Design review of the part built by this model. Coordinates are the model's own, in mm. Face numbers are marked on the shaded views. A direction names the side the tool comes from. Coordinates: 2 decimals unless noted, no trailing zeros. Loops run counter-clockwise (first coordinate to the right, second up) from the corner with the lowest first, then second, coordinate; pieces in that order, holes last. Notation, with made-up numbers: (83, 26) - (132, 26) arc R12 cw to (132, 45) - close; hole circle Ø8 at (50.5, 85.25). An arc over 180 degrees is marked (long way). Return JSON: item names as keys, results as strings. Group by question number.
from build123d import *

# Parameters (mm, degrees)
CROQUIS1_W              = 23
CROQUIS1_H              = 20
SALIENTE_EXTRUIR1_DEPTH = 9
CROQUIS2_W              = 6
CROQUIS2_H              = 12.95
CORTAR_EXTRUIR1_DEPTH   = 2
CROQUIS3_W              = 2.5
CROQUIS3_H              = 20
SALIENTE_EXTRUIR3_DEPTH = 15
CROQUIS4_R              = 1.85
CORTAR_EXTRUIR4_DEPTH   = 2.5
SALIENTE_EXTRUIR7_DEPTH = 2.5
CROQUIS7_W              = 10
CROQUIS7_H              = 15
CORTAR_EXTRUIR5_DEPTH   = 2.5
CROQUIS8_W              = 23
CROQUIS8_H              = 20
CORTAR_EXTRUIR6_DEPTH   = 3
CROQUIS9_W              = 2.5
CROQUIS9_H              = 10
CORTAR_EXTRUIR7_DEPTH   = 2
REDONDEO1_R             = 7
REDONDEO2_R             = 1


with BuildPart() as part:
    # Croquis1 → Saliente-Extruir1 (new body)
    with BuildSketch(Plane(origin=(0, 0, 0), x_dir=(1, 0, 0), z_dir=(0, 1, 0))):
        with Locations((11.5, -10)):
            Rectangle(CROQUIS1_W, CROQUIS1_H)
    extrude(amount=SALIENTE_EXTRUIR1_DEPTH)

    # Croquis2 → Cortar-Extruir1 (cut)
    with BuildSketch(Plane(origin=(0, 9, 0), x_dir=(1, 0, 0), z_dir=(0, 1, 0))):
        with Locations((20, -9.475)):
            Rectangle(CROQUIS2_W, CROQUIS2_H)
    extrude(amount=-CORTAR_EXTRUIR1_DEPTH, mode=Mode.SUBTRACT)

    # Croquis3 → Saliente-Extruir3 (add)
    with BuildSketch(Plane(origin=(0, 9, 0), x_dir=(1, 0, 0), z_dir=(0, 1, 0))):
        with Locations((1.25, -10)):
            Rectangle(CROQUIS3_W, CROQUIS3_H)
    extrude(amount=SALIENTE_EXTRUIR3_DEPTH)

    # Croquis4 → Cortar-Extruir4 (cut)
    with BuildSketch(Plane(origin=(2.5, 0, 0), x_dir=(0, 0, -1), z_dir=(1, 0, 0))):
        with Locations((-18, 15)):
            Circle(CROQUIS4_R)
    extrude(amount=-CORTAR_EXTRUIR4_DEPTH, mode=Mode.SUBTRACT)

    # Croquis6 → Saliente-Extruir7 (add)
    with BuildSketch(Plane(origin=(2.5, 0, 0), x_dir=(0, 0, -1), z_dir=(1, 0, 0))):
        with BuildLine():
            Line((-20, 19.418427322), (-20, 10.581572678))
            ThreePointArc((-20, 10.581572678), (-22.85, 15), (-20, 19.418427322))
        make_face()
    extrude(amount=-SALIENTE_EXTRUIR7_DEPTH)

    # Croquis7 → Cortar-Extruir5 (cut)
    with BuildSketch(Plane(origin=(2.5, 0, 0), x_dir=(0, 0, -1), z_dir=(1, 0, 0))):
        with Locations((-5, 16.5)):
            Rectangle(CROQUIS7_W, CROQUIS7_H)
    extrude(amount=-CORTAR_EXTRUIR5_DEPTH, mode=Mode.SUBTRACT)

    # Croquis8 → Cortar-Extruir6 (cut)
    with BuildSketch(Plane.XZ):
        with Locations((11.5, 10)):
            Rectangle(CROQUIS8_W, CROQUIS8_H)
    extrude(amount=-CORTAR_EXTRUIR6_DEPTH, mode=Mode.SUBTRACT)

    # Croquis9 → Cortar-Extruir7 (cut)
    with BuildSketch(Plane(origin=(0, 24, 0), x_dir=(1, 0, 0), z_dir=(0, 1, 0))):
        with Locations((1.25, -15)):
            Rectangle(CROQUIS9_W, CROQUIS9_H)
    extrude(amount=-CORTAR_EXTRUIR7_DEPTH, mode=Mode.SUBTRACT)

    # Redondeo1
    # the kernel refuses this fillet: 7 mm, written as the material it adds along each edge
    with BuildSketch(Plane(origin=(2.5, 9, 10), x_dir=(0, 0, -1), z_dir=(-1, 0, 0))) as redondeo1_piece_1:
        with BuildLine():
            CenterArc((REDONDEO1_R, -REDONDEO1_R), REDONDEO1_R, 90, 90)
            Line((0, -REDONDEO1_R), (0, 0))
            Line((0, 0), (REDONDEO1_R, 0))
        make_face()
    extrude(amount=2.5)
    with BuildSketch(Plane(origin=(2.5, 9, 10), x_dir=(1, 0, 0), z_dir=(0, 0, 1))) as redondeo1_piece_2_section:
        with BuildLine():
            CenterArc((REDONDEO1_R, REDONDEO1_R), REDONDEO1_R, 180, 90)
            Line((0, REDONDEO1_R), (0, 0))
            Line((0, 0), (REDONDEO1_R, 0))
        make_face()
    redondeo1_piece_2 = extrude(amount=10, mode=Mode.PRIVATE)
    redondeo1_piece_2 = redondeo1_piece_2 - Plane(origin=(2.5, 15, 18), x_dir=(0, 0, -1), z_dir=(1, 0, 0)) * Cylinder(1.85, 48, mode=Mode.PRIVATE)
    add(redondeo1_piece_2)
    with BuildSketch(Plane(origin=(2.5, 9, -7.5), x_dir=(1, 0, 0), z_dir=(0, 0, 1))) as redondeo1_piece_3_section:
        with BuildLine():
            CenterArc((REDONDEO1_R, REDONDEO1_R), REDONDEO1_R, 180, 90)
            Line((0, REDONDEO1_R), (0, 0))
            Line((0, 0), (REDONDEO1_R, 0))
        make_face()
    redondeo1_piece_3 = extrude(amount=45, mode=Mode.PRIVATE)
    redondeo1_piece_3 = split(redondeo1_piece_3, bisect_by=Plane(origin=(2.5, 9, 20), z_dir=(0, 0, 1)), keep=Keep.TOP, mode=Mode.PRIVATE)
    redondeo1_piece_3 = redondeo1_piece_3 & Plane(origin=(2.5, 15, 18), x_dir=(0, -0.9110159426851695, 0.4123711340206198), z_dir=(1, 0, 0)) * Cylinder(4.85, 118, mode=Mode.PRIVATE)
    add(redondeo1_piece_3)
    with BuildSketch(Plane(origin=(2.5, 9, -7.5), x_dir=(1, 0, 0), z_dir=(0, 0, 1))) as redondeo1_piece_4a_section:
        with BuildLine():
            CenterArc((REDONDEO1_R, REDONDEO1_R), REDONDEO1_R, 180, 90)
            Line((0, REDONDEO1_R), (0, 0))
            Line((0, 0), (REDONDEO1_R, 0))
        make_face()
    redondeo1_piece_4a = extrude(amount=27.5, mode=Mode.PRIVATE)
    redondeo1_piece_4a = split(redondeo1_piece_4a, bisect_by=Plane(origin=(2.5, 9, 0), z_dir=(0, 0, 1)), keep=Keep.TOP, mode=Mode.PRIVATE)
    redondeo1_piece_4a = split(redondeo1_piece_4a, bisect_by=Plane(origin=(2.5, 9, 10), z_dir=(0, 0, -1)), keep=Keep.TOP, mode=Mode.PRIVATE)
    with BuildSketch(Plane(origin=(20, 9, 10), x_dir=(0, 0, -1), z_dir=(-1, 0, 0))) as redondeo1_piece_4b_section:
        with BuildLine():
            CenterArc((REDONDEO1_R, -REDONDEO1_R), REDONDEO1_R, 90, 90)
            Line((0, -REDONDEO1_R), (0, 0))
            Line((0, 0), (REDONDEO1_R, 0))
        make_face()
    redondeo1_piece_4b = extrude(amount=20, mode=Mode.PRIVATE)
    redondeo1_piece_4b = split(redondeo1_piece_4b, bisect_by=Plane(origin=(2.5, 9, 10), z_dir=(1, 0, 0)), keep=Keep.TOP, mode=Mode.PRIVATE)
    redondeo1_piece_4b = split(redondeo1_piece_4b, bisect_by=Plane(origin=(17, 9, 10), z_dir=(-1, 0, 0)), keep=Keep.TOP, mode=Mode.PRIVATE)
    redondeo1_piece_4 = redondeo1_piece_4a & redondeo1_piece_4b
    add(redondeo1_piece_4)

    # Redondeo2
    redondeo2_edges = [part.edges().sort_by_distance(p)[0] for p in [
        (4.977657648, 10.656927883, 7.522342352),
        (0, 19, 10),
        (0, 11.050252532, 7.949747468),
        (7.147234739, 9.40723915, 20),
        (1.25, 22, 20),
        (0, 22, 15),
        (2.5, 22, 15),
        (2.5, 19, 10),
        (23, 9, 1.5),
        (23, 9, 17.975),
        (11.5, 9, 0),
        (0, 9, 1.5),
        (16.25, 9, 20),
    ]]
    fillet(redondeo2_edges, radius=REDONDEO2_R)


solid = part.part
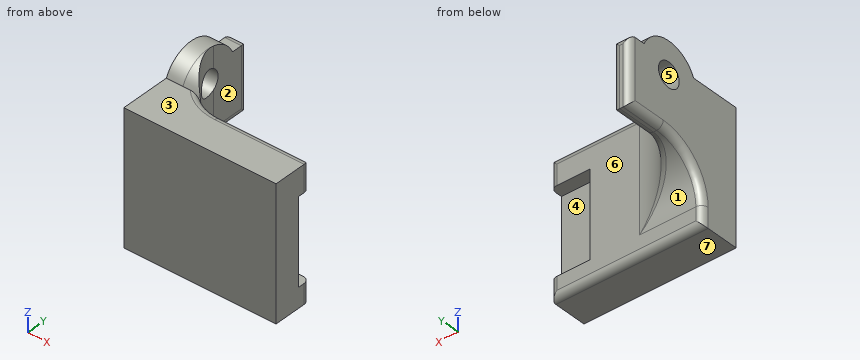
Item 1: Add section B-B (x = 20). State the section outline as (y, z) points.
Item 2: Add section A-A (z = 18). State the section outline as (x, y) points, then the cut area to 3 significant figures.
Item 3: To check wall thickness, follow line 1 (Y direction, x = 1.2, z = 18); line 2 (Y direction, x = 17, z = 17.5); line 3 (X direction, y = 7.75, z = 8.25). State the ranges of each line that lie inside material, in increasing order. Write a range as from..to.
Item 4: Add section C-C (y = 7.5). State the section outline as (x, z) points, then the cut area to 3 significant figures.
Item 5: For P1, Ø1.8, axis at x = 18.5, z = 6.5, coming from the +Y side; P2, Ø0.5, axis at x = 1.5, y = 20, coming from the +Z side; P3, Ø6, axis at x = 19.5, y = 11.5, coming from the +Z side, all flat-tipped, find the tip position at first contact; note any pin that passes through.
Item 6: Add section D-D (z = 13). State the section outline as (x, y) points.
Item 7: Draft analysis for pull direction Z (two halves, no side actions). For the marked faces 5, 6 and 7, state which applies: pulls with the +Z half, pulls with the -Z half, needs draft (parallel to the pull), parting line crosses it, or undercut.
Item 8: For the marked faces 1, 2, 3 and 4, list the 3-axis set-ups (+Z, -Z, +X, -X, +Y, -Y) from which the entire face can be reached by the end or side of a thin tool; tool diameter is ignored.
Answers below:
{
 "1": {"outline": "(3, 0) - (8, 0) arc R1 ccw to (9, 1) - (9, 3) - (7, 3) - (7, 15.95) - (9, 15.95) - (9, 19) arc R1 ccw to (8, 20) - (3, 20) - close"},
 "2": {"outline": "(0, 3) - (23, 3) - (23, 8) arc R1 ccw to (22, 9) - (9.5, 9) arc R7 cw to (3.11, 13.15) - (0, 13.15) - close; (0, 16.85) - (2.5, 16.85) - (2.5, 21) arc R1 ccw to (1.5, 22) - (1, 22) arc R1 ccw to (0, 21) - close", "area": "171 mm^2"},
 "3": {"line 1": "y = 3..13.15, 16.85..22", "line 2": "y = 3..9", "line 3": "x = 0..17"},
 "4": {"outline": "(0, 0) - (23, 0) - (23, 3) - (17, 3) - (17, 15.95) - (23, 15.95) - (23, 20) - (0, 20) - close", "area": "382 mm^2"},
 "5": {"P1": "stops at y = 7", "P2": "stops at z = 20", "P3": "stops at z = 19.87"},
 "6": {"outline": "(0, 3) - (23, 3) - (23, 7) - (17, 7) - (17, 9) - (9.5, 9) arc R7 cw to (2.5, 16) - (2.5, 21) arc R1 ccw to (1.5, 22) - (1, 22) arc R1 ccw to (0, 21) - close"},
 "7": {"face 5": "undercut", "face 6": "needs draft", "face 7": "pulls with the -Z half"},
 "8": {"face 1": "-Z, +X, -X, +Y", "face 2": "+Z, -Z, +X, +Y", "face 3": "+Z, +X, -X, -Y", "face 4": "+X, +Y"}
}
